Geometry: final body of the model. Coordinates: model frame, mm. Coordinates: 2 decimals unless noted, no trailing zeros. Loops run counter-clockwise (first coordinate to the right, second up) from the corner with the lowest first, then second, coordinate; pieces in that order, holes last. Notation, with made-up numbers: (50.5, 54.25) -> (98.5, 54.25) arc R18 ccw to (98.5, 63.25) -> close; hole circle Ø3 at (8.25, 22). An arc over 180 degrees is marked (long way). One line per item, written item: value. Start each with the question number.
Item 1: Contact query for flat-ended pins moving along their axis: pin 1 Ø1.7 at (x, y) = (-24.5, 1.5) entering from +Z; pin 2 Ø8 at (x, z) = (-6, -7.5) entering from +Y. Output: stop coordinate, or through.
Item 2: Section query A-A on y = -1.6. Return loops of the section in (x, z).
Item 3: Section query D-D on y = 1.9. Return loops of the section in (x, z), then the cut area to 3 significant figures.
Item 4: Section query B-B on x = -8.5. Return loops of the section in (y, z).
Item 5: Ray query, probe 1 along Z at (x, y) = (-26.5, 2.55); probe 2 along X at (y, z) = (-0.2, -3.75); probe 3 along X at (y, z) = (2.65, 3.75). Return the intervals inside material, ascending. Write a range as from..to.
Item 6: Section query C-C on z = -2. Return loops of the section in (x, y), then the cut area to 3 significant figures.
from build123d import *

# Parameters (mm, degrees)
PAD_DEPTH    = 3.9
SKETCH001_R  = 2.9
PAD001_DEPTH = 11


with BuildPart() as part:
    # Sketch → Pad (new body, symmetric)
    with BuildSketch(Plane.XY):
        with BuildLine():
            ThreePointArc((-1.2e-05, -2.9), (2.9, 0), (-1.2e-05, 2.9))
            Line((-1.2e-05, 2.9), (-32.917675, 2.9))
            Line((-32.917675, -2.9), (-32.917675, 2.9))
            Line((-1.2e-05, -2.9), (-32.917675, -2.9))
        make_face()
    extrude(amount=PAD_DEPTH, both=True)

    # Sketch001 → Pad001 (join, symmetric)
    with BuildSketch(Plane.XY):
        Circle(SKETCH001_R)
    extrude(amount=PAD001_DEPTH, both=True)


solid = part.part
Reply:
1. pin 1: stops at z = 3.9
1. pin 2: stops at y = 2.9
2. outline: (-32.92, -3.9) -> (-2.42, -3.9) -> (-2.42, -11) -> (2.42, -11) -> (2.42, 11) -> (-2.42, 11) -> (-2.42, 3.9) -> (-32.92, 3.9) -> close
3. outline: (-32.92, -3.9) -> (-2.19, -3.9) -> (-2.19, -11) -> (2.19, -11) -> (2.19, 11) -> (-2.19, 11) -> (-2.19, 3.9) -> (-32.92, 3.9) -> close
3. area: 336 mm²
4. outline: (-2.9, -3.9) -> (2.9, -3.9) -> (2.9, 3.9) -> (-2.9, 3.9) -> close
5. probe 1: z = -3.9..3.9
5. probe 2: x = -32.92..2.89
5. probe 3: x = -32.92..1.18
6. outline: (-32.92, -2.9) -> (0, -2.9) arc R2.9 ccw to (0, 2.9) -> (-32.92, 2.9) -> close
6. area: 204 mm²
